Verification items for this drawing (mm, ordinates from the low corner). A direction names the side the tool comes from. Give positions to 0.01 mm unless a question says otherwise; leave off trailing zeros. Loops run counter-clockwise (first coordinate to the right, second up) from the corner with the lowest first, then second, coordinate; pieces in that order, holes last. Notation, with made-up numbers: M 46,44.25 L 56,44.25 A10 cw 56,57.25 Z; hole C 59.25,1 d4. An arc over 180 degrees is marked long. Write each question's results on one line, items separated by ' | '. Start each with the question number.
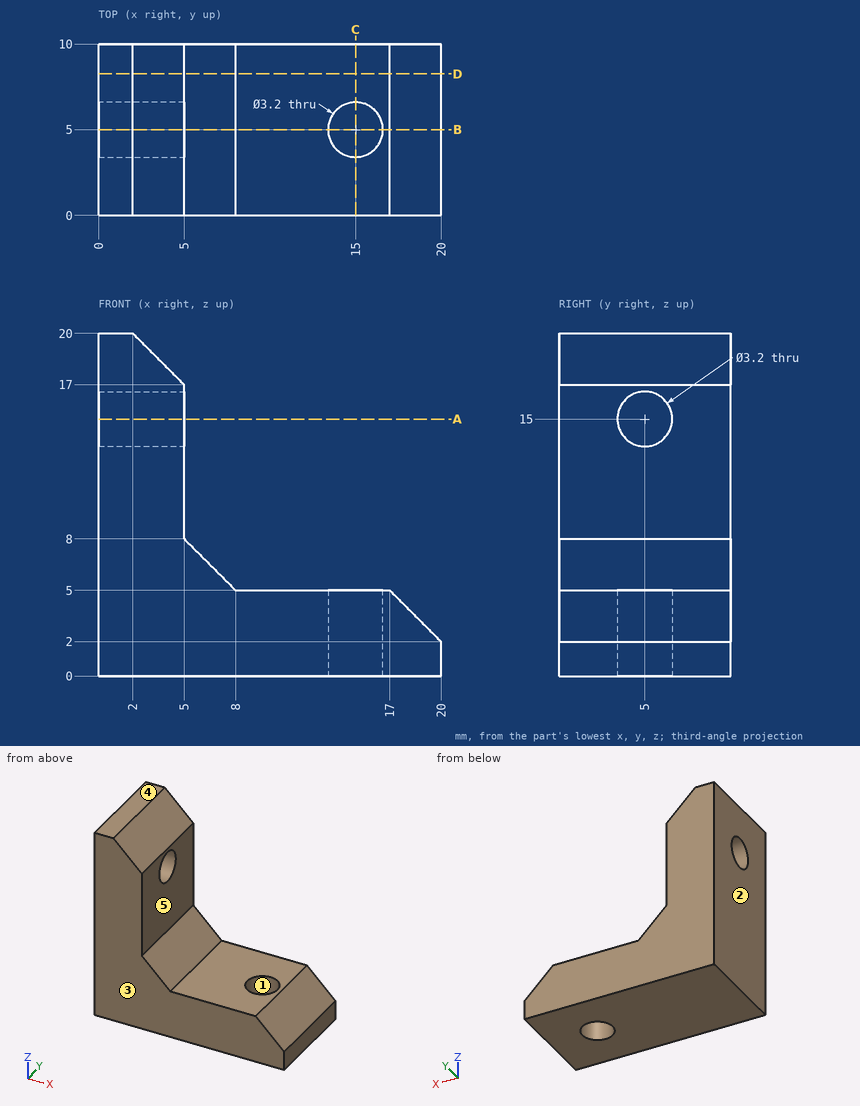
1. Section check D-D, the plane y = 8.25. Record the boundary of the cut face in (x, z).
2. Thickness scan on probe 1 along Y at (x, z) = (15, 1.25); probe 2 along X at (y, z) = (8.5, 10); probe 3 along Z at (x, y) = (1.95, 5). Record the ranges inside material, lowest first.
3. Section check C-C, the plane x = 15. Record the boundary of the cut face in (y, z), plus the area to 3 significant figures.
4. Set-up check for the marked faces 4 and 5: record each of +Z, -Z, +X, -X, +Y, -Y from which the full face is reachable in a straight line by a thin tool's end or side.
5. Section check B-B, the plane y = 5. Record the boundary of the cut face in (x, z), plus the area to 4 significant figures.
6. Release check for a two-part mould opening along Y. For the marked faces 1, 2 and 3 record: released by +Y, released by -Y, zero draft, split by the parting line, or undercut.
7. Depth check by flat-ended pin: pin 1 Ø4.5 at (x, y) = (12, 6) entering from +Z; pin 2 Ø5 at (y, z) = (7.5, 8) entering from +X. Enter the tip coordinate at first touch or a pass-through.
8. Section check A-A, the plane z = 15. Record the boundary of the cut face in (x, y), plus the area to 3 significant figures.
Filled sheet:
1) outline: M 0,0 L 20,0 L 20,2 L 17,5 L 8,5 L 5,8 L 5,17 L 2,20 L 0,20 Z
2) probe 1: 0 to 3.4, 6.6 to 10 | probe 2: 0 to 5 | probe 3: 0 to 13.4, 16.6 to 20
3) outline: M 0,0 L 3.4,0 L 3.4,5 L 0,5 Z; M 6.6,0 L 10,0 L 10,5 L 6.6,5 Z | area: 34.0 mm2
4) face 4: +Z, +X, -X, +Y, -Y | face 5: +Z, +X, +Y, -Y
5) outline: M 0,0 L 13.4,0 L 13.4,5 L 8,5 L 5,8 L 5,13.4 L 0,13.4 Z; M 0,16.6 L 5,16.6 L 5,17 L 2,20 L 0,20 Z; M 16.6,0 L 20,0 L 20,2 L 17,5 L 16.6,5 Z | area: 138.5 mm2
6) face 1: undercut | face 2: zero draft | face 3: released by -Y
7) pin 1: z = 5 | pin 2: x = 7.5
8) outline: M 0,0 L 5,0 L 5,3.4 L 0,3.4 Z; M 0,6.6 L 5,6.6 L 5,10 L 0,10 Z | area: 34.0 mm2
